from build123d import *

# Parameters (mm, degrees)
F0_W     = 150.0124
F0_H     = 75.9968
F0_R     = 2.5019
F1_DEPTH = 11.9888


with BuildPart() as f1:
    # F0 (on Front) → F1 (new body)
    with BuildSketch(Plane.XZ):
        Rectangle(F0_W, F0_H)
        with Locations((-65.567933, -27.9908)):
            Circle(F0_R, mode=Mode.SUBTRACT)
        with Locations((-52.867933, -27.9908)):
            Circle(F0_R, mode=Mode.SUBTRACT)
        with Locations((-22.808934, -27.9908)):
            Circle(F0_R, mode=Mode.SUBTRACT)
        with Locations((-10.108934, -27.9908)):
            Circle(F0_R, mode=Mode.SUBTRACT)
        with Locations((-65.567933, 27.9908)):
            Circle(F0_R, mode=Mode.SUBTRACT)
        with Locations((-52.867933, 27.9908)):
            Circle(F0_R, mode=Mode.SUBTRACT)
        with Locations((-22.808934, 27.9908)):
            Circle(F0_R, mode=Mode.SUBTRACT)
        with Locations((-10.108934, 27.9908)):
            Circle(F0_R, mode=Mode.SUBTRACT)
        with Locations((51.660687, 22.5044)):
            Circle(F0_R, mode=Mode.SUBTRACT)
        with Locations((71.980687, 22.5044)):
            Circle(F0_R, mode=Mode.SUBTRACT)
        with Locations((51.660687, 32.448623)):
            Circle(F0_R, mode=Mode.SUBTRACT)
        with Locations((71.980687, 32.623451)):
            Circle(F0_R, mode=Mode.SUBTRACT)
    extrude(amount=F1_DEPTH)


solid = f1.part
Could you check a few things on this model? Use its own coordinates, in mm. Give positions to 0.01 mm unless a question says otherwise; leave off trailing zeros. Order: outer loops, then holes, each group sorted by start corner. A loop starts at its lowest first (then second) coordinate and runs counter-clockwise, first axis right, second up. Notation, with made-up numbers: (74.25, -31.5) -> (127.25, -31.5) arc R7 cw to (127.25, -21.5) -> close; hole circle Ø4 at (30, -4.75). An arc over 180 degrees is marked (long way). Return JSON: item names as keys, results as strings.
1. Thinking about a two-plate mould opening in Z: for faces 1 (the flat face through (-1, -6, -37.998)), 2 (the flat face through (-75.006, -6, -1)), 3 (the cylindrical face through (69.48, -5.91, 22.61)), 4 (the cylindrical face through (-53.41, -5.91, -30.433)), which applies, pulls with the +Z half, pulls with the -Z half, needs draft (parallel to the pull), parting line crosses it, or undercut?
Answer list:
{"face 1": "pulls with the -Z half", "face 2": "needs draft", "face 3": "undercut", "face 4": "undercut"}
2. For pin 1 Ø4.5 at (x, z) = (-52.87, 27.99) entering from +Y; pin 2 Ø5 at (x, z) = (-11, -20.5) entering from +Y, each with a flat end and sliding along its axis, tell me the tip position at first contact or that it passes through.
Answer list:
{"pin 1": "passes through", "pin 2": "stops at y = 0"}
3. Imagine slicing it at A-A on x = -23. List the corners of the cut face in (y, z) for me.
Answer list:
{"outline": "(-11.99, -38) -> (0, -38) -> (0, -30.49) -> (-11.99, -30.49) -> close; (-11.99, -25.5) -> (0, -25.5) -> (0, 25.5) -> (-11.99, 25.5) -> close; (-11.99, 30.49) -> (0, 30.49) -> (0, 38) -> (-11.99, 38) -> close"}
4. Imagine slicing it at C-C on x = -66. List the corners of the cut face in (y, z) for me, then the cut area to 3 significant figures.
Answer list:
{"outline": "(-11.99, -38) -> (0, -38) -> (0, -30.46) -> (-11.99, -30.46) -> close; (-11.99, -25.53) -> (0, -25.53) -> (0, 25.53) -> (-11.99, 25.53) -> close; (-11.99, 30.46) -> (0, 30.46) -> (0, 38) -> (-11.99, 38) -> close", "area": "793 mm2"}
5. I need wall thicknesses on line 1 (X direction, y = -3.5, z = 32.5); line 2 (X direction, y = -9.25, z = 23.5); line 3 (X direction, y = -3.25, z = 28.5). Which ranges of each line are inside material? Lowest first, please. Write a range as from..to.
Answer list:
{"line 1": "x = -75.01..49.16, 54.16..69.48, 74.48..75.01", "line 2": "x = -75.01..49.37, 53.96..69.69, 74.28..75.01", "line 3": "x = -75.01..-68.02, -63.12..-55.32, -50.42..-25.26, -20.36..-12.56, -7.66..75.01"}
6. Imagine slicing it at B-B on y = -10. Give the number of separate pieces and of enclosed holes in the cut face, then the cut area to 3 significant figures.
Answer list:
{"separate pieces": "1", "enclosed holes": "12", "area": "11,200 mm2"}
